```python
from build123d import *

# Parameters (mm, degrees)
F0_R     = 52.324
F0_R_2   = 1.5875
F1_DEPTH = 2.54
F2_R     = 49.276
F2_R_2   = 45.2755
F3_DEPTH = 1.27
F4_R     = 8.255
F5_DEPTH = 2.541


with BuildPart() as f1:
    # F0 (on Top) → F1 (new body)
    with BuildSketch(Plane.XY):
        Circle(F0_R)
        Circle(F0_R_2, mode=Mode.SUBTRACT)
    extrude(amount=F1_DEPTH)

    # F2 (on face) → F3 (cut)
    with BuildSketch(Plane.XY.offset(2.54)):
        Circle(F2_R)
        Circle(F2_R_2, mode=Mode.SUBTRACT)
    extrude(amount=-F3_DEPTH, mode=Mode.SUBTRACT)

    # F4 (on face) → F5 (cut, through all)
    with BuildSketch(Plane.XY.offset(2.54)):
        with Locations((0, -31.75)):
            Circle(F4_R)
    extrude(amount=-F5_DEPTH, mode=Mode.SUBTRACT)


solid = f1.part
```
Could you check a few things on this model? Use its own coordinates, in mm. A direction names the side the tool comes from. Round coordinates to 2 decimals unless told otherwise and drop trailing zeros. Loops run counter-clockwise (first coordinate to the right, second up) from the corner with the lowest first, then second, coordinate; pieces in that order, holes last.
Q1. On a 3-axis mill with a long thin cutter (end or side, diameter ignored), from which of +Z, -Z, +X, -X, +Y, -Y can I reach the whole of each face in a straight line? I mean faces 1 (the flat face through (39, -31, 2.54)), 2 (the flat face through (22, -40, 1.27)). Say none if no direction works.
Q2. I want a section at B-B (y = 0). Write out the boundary of the cut face in (x, z), and give its area (3 significant figures).
Q3. Please list where these lines run through material, in increasing order: L1, parallel to Y at x = 0, z = 1.1 (1 decimal); L2, parallel to Y at x = 19.5, z = 1.8; L3, parallel to X at y = -26, z = 2.3.
Q4. I want a section at D-D (y = -18). Write out the boundary of the cut face in (x, z), and give its area (3 significant figures).
Q5. Thinking about a two-plate mould opening in Y: for faces 3 (the cylindrical face through (-6.81, 51.88, 1.25)), 4 (the cylindrical face through (-10.7, -48.1, 1.9)), 5 (the flat face through (9, 1, 2.54)), which applies, pulls with the +Y half, pulls with the -Y half, needs draft (parallel to the pull), parting line crosses it, or undercut?
Q6. I want a section at A-A (x = 0). Write out the boundary of the cut face in (y, z) (1 decimal), and give its area (3 significant figures).
Q7. I want a section at C-C (x = -32.5). Write out the boundary of the cut face in (y, z).
Q8. For P1, Ø3, axis at x = 0, y = 0, coming from the +Z side; P2, Ø3, axis at x = 27.5, y = 7, coming from the -Z side; P3, Ø1.5, axis at x = 15.5, z = 0.5, coming from the -Y side, each with a flat end and sliding along its axis, tell me the tip position at first contact or that it passes through.
Answer below:
1. face 1: +Z, +X, -X, +Y, -Y
1. face 2: +Z
2. outline: (-52.32, 0) - (-1.59, 0) - (-1.59, 2.54) - (-45.28, 2.54) - (-45.28, 1.27) - (-49.28, 1.27) - (-49.28, 2.54) - (-52.32, 2.54) - close; (1.59, 0) - (52.32, 0) - (52.32, 2.54) - (49.28, 2.54) - (49.28, 1.27) - (45.28, 1.27) - (45.28, 2.54) - (1.59, 2.54) - close
2. area: 248 mm2
3. L1: y = -52.3 to -40, -23.5 to -1.6, 1.6 to 52.3
3. L2: y = -48.55 to -45.25, -40.86 to 40.86, 45.25 to 48.55
3. L3: x = -45.41 to -41.86, -37.07 to -5.92, 5.92 to 37.07, 41.86 to 45.41
4. outline: (-49.13, 0) - (49.13, 0) - (49.13, 2.54) - (45.87, 2.54) - (45.87, 1.27) - (41.54, 1.27) - (41.54, 2.54) - (-41.54, 2.54) - (-41.54, 1.27) - (-45.87, 1.27) - (-45.87, 2.54) - (-49.13, 2.54) - close
4. area: 239 mm2
5. face 3: parting line crosses it
5. face 4: undercut
5. face 5: needs draft
6. outline: (-52.3, 0) - (-40, 0) - (-40, 2.5) - (-45.3, 2.5) - (-45.3, 1.3) - (-49.3, 1.3) - (-49.3, 2.5) - (-52.3, 2.5) - close; (-23.5, 0) - (-1.6, 0) - (-1.6, 2.5) - (-23.5, 2.5) - close; (1.6, 0) - (52.3, 0) - (52.3, 2.5) - (49.3, 2.5) - (49.3, 1.3) - (45.3, 1.3) - (45.3, 2.5) - (1.6, 2.5) - close
6. area: 206 mm2
7. outline: (-41.01, 0) - (41.01, 0) - (41.01, 2.54) - (37.04, 2.54) - (37.04, 1.27) - (31.52, 1.27) - (31.52, 2.54) - (-31.52, 2.54) - (-31.52, 1.27) - (-37.04, 1.27) - (-37.04, 2.54) - (-41.01, 2.54) - close
8. P1: passes through
8. P2: stops at z = 0
8. P3: stops at y = -50.2
